```python
from build123d import *

# Parameters (mm, degrees)
SKETCH_1_W                   = 34
SKETCH_1_H                   = 30
SKETCH_1_R                   = 5.15
EXTRUDE_1_DEPTH              = 30
HOLE_WIZARD_M4_1_D           = 3.3
HOLE_WIZARD_M4_1_DEPTH       = 12.1
HOLE_WIZARD_M4_1_CSINK_D     = 4.05
HOLE_WIZARD_M4_1_CSINK_ANGLE = 90
HOLE_WIZARD_M4_1_TIP         = 0.991420021
HOLE_WIZARD_M3_1_D           = 2.5
HOLE_WIZARD_M3_1_DEPTH       = 7.5
HOLE_WIZARD_M3_1_CSINK_D     = 3.05
HOLE_WIZARD_M3_1_CSINK_ANGLE = 90
HOLE_WIZARD_M3_1_TIP         = 0.751075774


with BuildPart() as part:
    # 草图1 → 凸台-拉伸1 (new body)
    with BuildSketch(Plane.XY):
        with Locations((0, 1)):
            Rectangle(SKETCH_1_W, SKETCH_1_H)
        Circle(SKETCH_1_R, mode=Mode.SUBTRACT)
    extrude(amount=EXTRUDE_1_DEPTH)

    # M4 螺纹孔1
    with Locations(Plane(origin=(0, 16, 0), x_dir=(1, 0, 0), z_dir=(0, 1, 0))):
        with Locations((-12, -5), (12, -5), (-12, -25), (12, -25)):
            CounterSinkHole(HOLE_WIZARD_M4_1_D / 2, HOLE_WIZARD_M4_1_CSINK_D / 2, depth=HOLE_WIZARD_M4_1_DEPTH, counter_sink_angle=HOLE_WIZARD_M4_1_CSINK_ANGLE)
            with Locations((0, 0, -(HOLE_WIZARD_M4_1_DEPTH + HOLE_WIZARD_M4_1_TIP / 2))):  # 118° drill point
                Cone(0, HOLE_WIZARD_M4_1_D / 2, HOLE_WIZARD_M4_1_TIP, mode=Mode.SUBTRACT)

    # M3 螺纹孔1
    with Locations(Plane.XY.offset(30)):
        with Locations((0, 8), (-8, 0), (8, 0), (0, -8)):
            CounterSinkHole(HOLE_WIZARD_M3_1_D / 2, HOLE_WIZARD_M3_1_CSINK_D / 2, depth=HOLE_WIZARD_M3_1_DEPTH, counter_sink_angle=HOLE_WIZARD_M3_1_CSINK_ANGLE)
            with Locations((0, 0, -(HOLE_WIZARD_M3_1_DEPTH + HOLE_WIZARD_M3_1_TIP / 2))):  # 118° drill point
                Cone(0, HOLE_WIZARD_M3_1_D / 2, HOLE_WIZARD_M3_1_TIP, mode=Mode.SUBTRACT)


solid = part.part
```
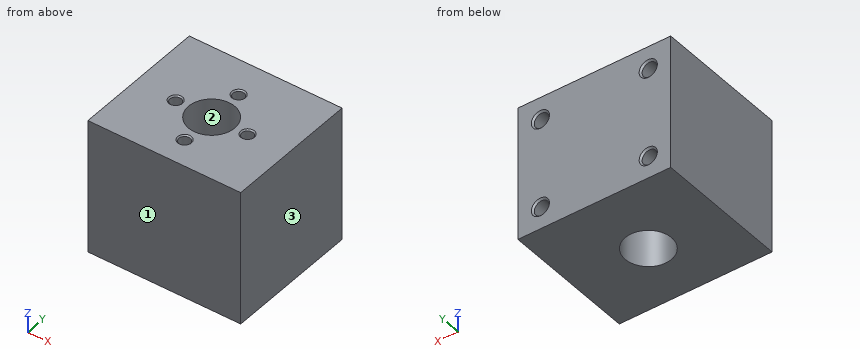
Model file for the job. Use its own axes, mm. Face numbers are marked on the shaded views. Round coordinates to 2 decimals unless told otherwise and drop trailing zeros. Order: outer loops, then holes, each group sorted by start corner. A loop starts at its lowest first (then second) coordinate and runs counter-clockwise, first axis right, second up. Notation, with made-up numbers: (15, 3.5) -> (63, 3.5) arc R29 ccw to (63, 38.5) -> close; hole circle Ø1 at (31.25, -35.75). An arc over 180 degrees is marked (long way). Use one line per item in the form item = value.
Item 1: Flat gauge pins, fed straight in: pin 1 Ø8 at (x, y) = (0, 0) entering from +Z; pin 2 Ø2 at (x, y) = (-8, 0) entering from +Z; pin 3 Ø3 at (x, y) = (0, -8) entering from +Z (3 decimals); pin 4 Ø4 at (x, z) = (-12, 5) entering from +Y (3 decimals). Where does each tip first touch, or does it go through?
Returned:
pin_1 = through
pin_2 = 22.35
pin_3 = 29.975
pin_4 = 15.975
Item 2: Cut at C-C, the plane z = 20.5. Write the cut outline in (x, y).
Returned:
outline = (-17, -14) -> (17, -14) -> (17, 16) -> (-17, 16) -> close; hole circle Ø10.3 at (0, 0)
Item 3: Drill centre lines: line 1 (Y direction, x = 0, z = 27.5); line 2 (Z direction, x = -12, y = 12.5); line 3 (X direction, y = 11.5, z = 25). Where is each one in solid material? Low to high.
Returned:
line_1 = -14 to -9.25, -6.75 to -5.15, 5.15 to 6.75, 9.25 to 16
line_2 = 0 to 3.35, 6.65 to 23.35, 26.65 to 30
line_3 = -17 to -13.65, -10.35 to 10.35, 13.65 to 17
Item 4: Cut at A-A, the plane y = 12.75. Write the cut outline in (x, z), and give its area (3 significant figures).
Returned:
outline = (-17, 0) -> (17, 0) -> (17, 30) -> (-17, 30) -> close; hole circle Ø3.3 at (-12, 5); hole circle Ø3.3 at (-12, 25); hole circle Ø3.3 at (12, 5); hole circle Ø3.3 at (12, 25)
area = 986 mm^2
Item 5: Cut at B-B, the plane x = -3. Write the cut outline in (y, z), and give its area (3 significant figures).
Returned:
outline = (-14, 0) -> (-4.19, 0) -> (-4.19, 30) -> (-14, 30) -> close; (4.19, 0) -> (16, 0) -> (16, 30) -> (4.19, 30) -> close
area = 649 mm^2
Item 6: Pull direction Y, two halves, no side cores. Call the marked faces 1, 2 and 3: released by +Y, released by -Y, zero draft, split by the parting line, or undercut.
Returned:
face_1 = released by -Y
face_2 = undercut
face_3 = zero draft
